The figure shows three views and two pictorial views of one solid part (mm, origin at its lowest corner). Answer the questions. A direction names the side the tool comes from. Give positions to 0.01 mm unless a question says otherwise; leave off trailing zeros. Order: outer loops, then holes, each group sorted by start corner. A loop starts at its lowest first (then second) coordinate and runs counter-clockwise, first axis right, second up. Notation, with made-up numbers: M 81.5,49 L 121.5,49 A17 cw 121.5,62 Z; hole C 25.25,-9.75 d5. An arc over 180 degrees is marked long. Write item = value, one per line. Start each with the question number.
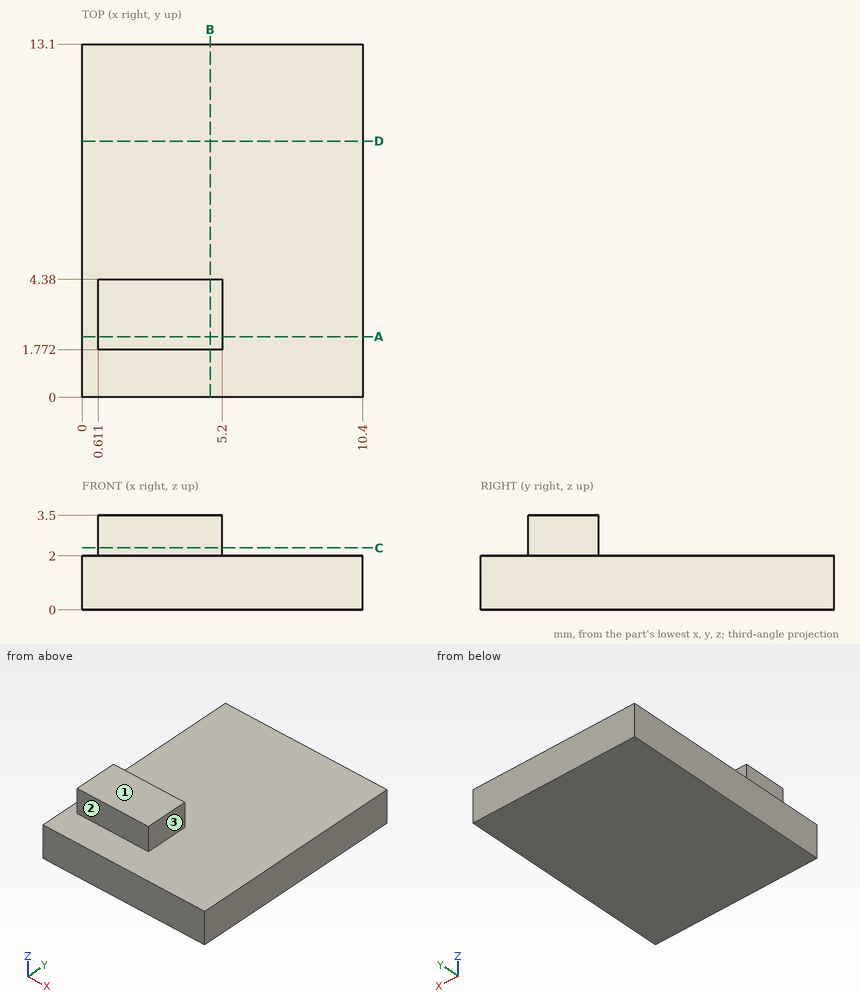
1) Find section D-D on y = 9.5. Determine the outline of the cut face in (x, z), plus the area to 3 significant figures.
2) Find section A-A on y = 2.25. Determine the outline of the cut face in (x, z).
3) For the marked faces 1, 2 and 3, determine the directions among +Z, -Z, +X, -X, +Y, -Y from which every point of the face is accessible in a straight line to the end or side of a thin tool.
4) Each of these flat-tipped pins is pushed along its axis until it touches: P1, Ø4, axis at x = 7.5, y = 10, coming from the +Z side; P2, Ø0.8, axis at y = 3.5, z = 3, coming from the -X side; P3, Ø1.2, axis at y = 3, z = 3, coming from the +X side. Where does it stop, or does it pass through?
5) Find the intervals of material crossed by probe 1 along Z at (x, y) = (4.25, 7.25); probe 2 along Y at (x, z) = (3.75, 3.2); probe 3 along X at (y, z) = (4.25, 2.1), in increasing order. Write a range as [from, to].
6) Find section B-B on x = 4.75. Determine the outline of the cut face in (y, z), plus the area to 3 significant figures.
7) Find section C-C on z = 2.3. Determine the outline of the cut face in (x, y), plus the area to 3 significant figures.
Numbers:
q1.outline = M 0,0 L 10.4,0 L 10.4,2 L 0,2 Z
q1.area = 20.8 mm2
q2.outline = M 0,0 L 10.4,0 L 10.4,2 L 5.2,2 L 5.2,3.5 L 0.61,3.5 L 0.61,2 L 0,2 Z
q3.face_1 = +Z, +X, -X, +Y, -Y
q3.face_2 = +Z, +X, -X, -Y
q3.face_3 = +Z, +X, +Y, -Y
q4.P1 = 2
q4.P2 = 0.61
q4.P3 = 5.2
q5.probe_1 = [0, 2]
q5.probe_2 = [1.77, 4.38]
q5.probe_3 = [0.61, 5.2]
q6.outline = M 0,0 L 13.1,0 L 13.1,2 L 4.38,2 L 4.38,3.5 L 1.77,3.5 L 1.77,2 L 0,2 Z
q6.area = 30.1 mm2
q7.outline = M 0.61,1.77 L 5.2,1.77 L 5.2,4.38 L 0.61,4.38 Z
q7.area = 12.0 mm2
